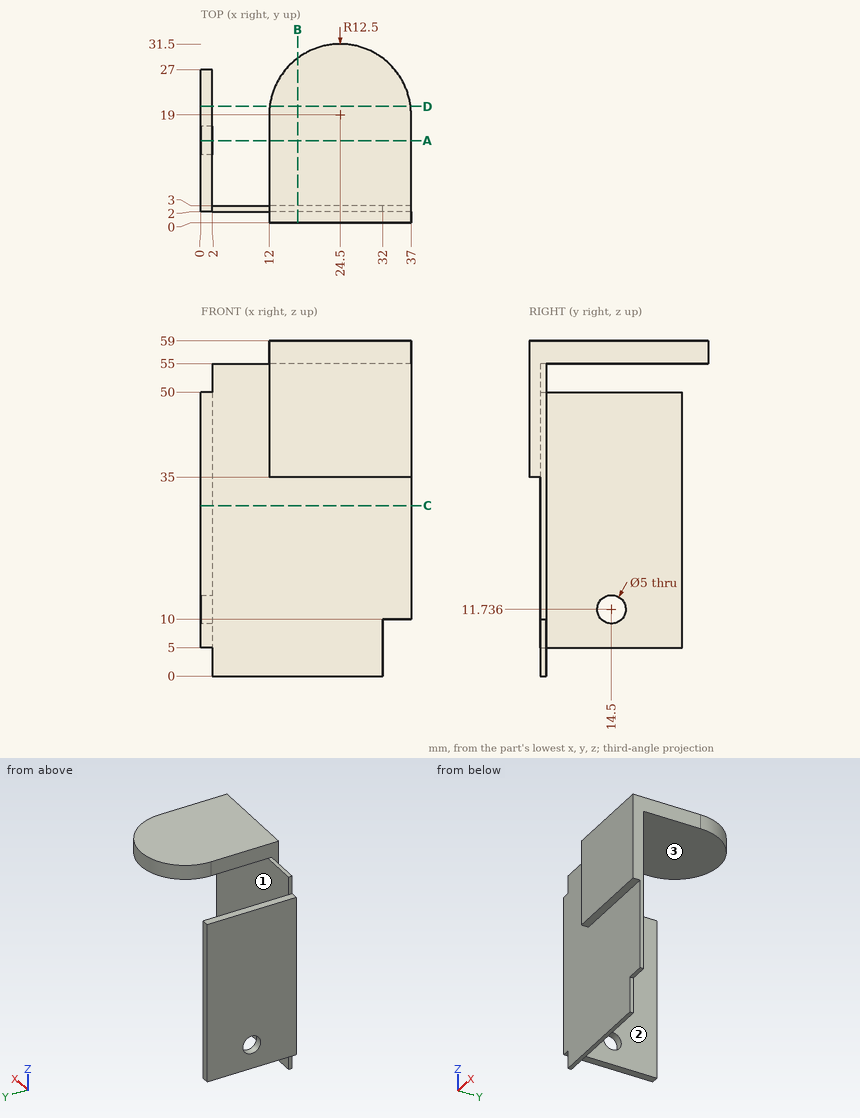
Geometry: see drawing. Coordinates: mm, zero at the bounding-box minimum. A direction names the side the tool comes from. Round coordinates to 2 decimals unless told otherwise and drop trailing zeros. Loops run counter-clockwise (first coordinate to the right, second up) from the corner with the lowest first, then second, coordinate; pieces in that order, holes last. Notation, with made-up numbers: (-33.75, 7.25) - (3.25, 7.25) arc R27 cw to (3.25, 39.25) - close; hole circle Ø2 at (0.25, 86). An arc over 180 degrees is marked (long way). One line per item, written item: value. Start each with the question number.
(1) Section A-A, the plane y = 14.5. Return loops of the section in (x, z), plus the area to 3 significant figures.
(2) Ray query, line 1 (Y direction, x = 23.5, z = 8); line 2 (X direction, y = 9.5, z = 22); line 3 (Z direction, x = 26.5, y = 23). Return the intervals inside material, ascending. Write a range as [from, to].
(3) Contact query for flat-ended pins moving along their axis: P1, Ø1.5, axis at x = 20, z = 36, coming from the +Y side; P2, Ø3, axis at y = 18, z = 23.5, coming from the -X side; P3, Ø3, axis at x = 10, y = 12, coming from the +Z side; P4, Ø2, axis at x = 21, z = 7.5, coming from the -Y side. Output: stop coordinate, or through.
(4) Access query for the marked faces 1, 2 and 3. Directions: +Z, -Z, +X, -X, +Y, -Y. A direction counts if a zero-diameter tool reaches every point of the face in a straight line with its end or side. Return the directions, or none.
(5) Section B-B, the plane x = 17. Return loops of the section in (y, z).
(6) Section C-C, the plane z = 30. Return loops of the section in (x, y).
(7) Section D-D, the plane y = 20.5. Return loops of the section in (x, z), plus the area to 3 significant figures.
Results below:
1. outline: (0, 5) - (2, 5) - (2, 9.24) - (0, 9.24) - close; (0, 14.24) - (2, 14.24) - (2, 50) - (0, 50) - close; (12, 55) - (37, 55) - (37, 59) - (12, 59) - close
1. area: 180 mm^2
2. line 1: [2, 3]
2. line 2: [0, 2]
2. line 3: [55, 59]
3. P1: y = 3
3. P2: x = 0
3. P3: through
3. P4: y = 2
4. face 1: -Z, +X, +Y
4. face 2: +Z, -Z, +X, +Y
4. face 3: -Z, +X, -X, +Y
5. outline: (0, 35) - (2, 35) - (2, 0) - (3, 0) - (3, 55) - (29, 55) - (29, 59) - (0, 59) - close
6. outline: (0, 2) - (37, 2) - (37, 3) - (2, 3) - (2, 27) - (0, 27) - close
7. outline: (0, 5) - (2, 5) - (2, 50) - (0, 50) - close; (12.09, 55) - (36.91, 55) - (36.91, 59) - (12.09, 59) - close
7. area: 189 mm^2
